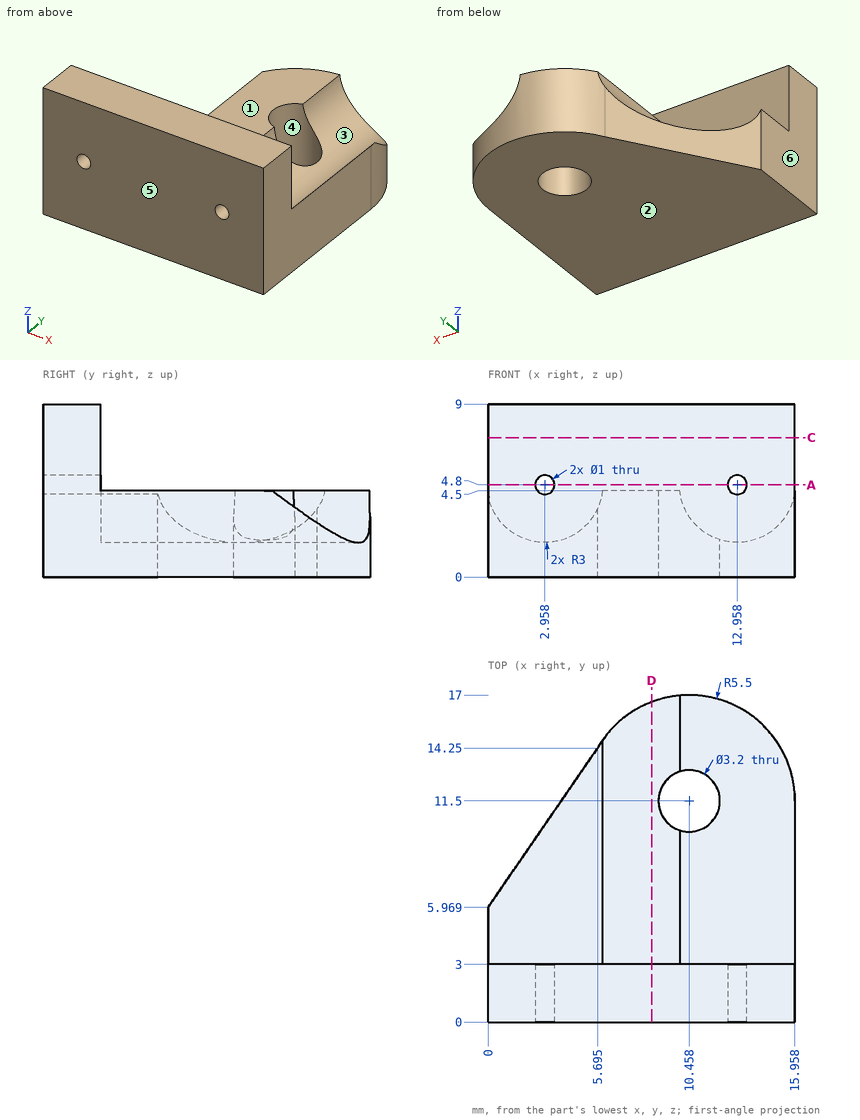
Study the drawing (mm; zero at the part's minimum x, y, z) and answer. A direction names the side the tool comes from. Round coordinates to 2 decimals unless told otherwise and drop trailing zeros. Order: outer loops, then holes, each group sorted by start corner. A loop starts at its lowest first (then second) coordinate and runs counter-clockwise, first axis right, second up. Notation, with made-up numbers: (36, 45) - (83, 45) arc R28 cw to (83, 80) - close; hole circle Ø9 at (-4, 35). An arc over 180 degrees is marked (long way). Use one line per item in the form item = value. Start each with the question number.
(1) A flat-ended cylindrical pin translates along its axis: pin 1 Ø1.2 at (x, y) = (7.5, 7.5) entering from +Z. Find the tip coordinate at first contact, or state that the pin passes through.
(2) For the marked faces 1, 2 and 3, determine the directions among +Z, -Z, +X, -X, +Y, -Y from which every point of the face is accessible in a straight line to the end or side of a thin tool.
(3) The part is cut by section D-D (x = 8.5). Give the vertices of the cut face in (y, z), then the cut area to 3 significant figures.
(4) The part is cut by section C-C (z = 7.25). Give the vertices of the cut face in (x, y).
(5) Determine the mould class of the marked faces 4, 5 and 6 for opening direction Y: +Y half, -Y half, draft (parallel to the pull), parting line (faces both ways), or undercut.
(6) The part is cut by section A-A (z = 4.8). Give the vertices of the cut face in (x, y).
(7) Find the intervals of material crossed by line 1 along Y through (x, z) = (4.25, 4); line 2 along Z through (x, y) = (6, 9); line 3 along Z through (x, y) = (13, 15), in increasing order. Write a range as from..to.
Checked values:
q1.pin_1 = 4.5
q2.face_1 = +Z, +X, -X, +Y
q2.face_2 = -Z, +X, -X, +Y, -Y
q2.face_3 = +Z, +Y
q3.outline = (0, 0) - (16.64, 0) - (16.64, 4.5) - (3, 4.5) - (3, 9) - (0, 9) - close
q3.area = 88.4 mm^2
q4.outline = (0, 0) - (15.96, 0) - (15.96, 3) - (0, 3) - close
q5.face_4 = undercut
q5.face_5 = -Y half
q5.face_6 = draft
q6.outline = (0, 0) - (2.46, 0) - (2.46, 3) - (0, 3) - close; (3.46, 0) - (12.46, 0) - (12.46, 3) - (3.46, 3) - close; (13.46, 0) - (15.96, 0) - (15.96, 3) - (13.46, 3) - close
q7.line_1 = 0..3
q7.line_2 = 0..4.5
q7.line_3 = 0..1.8
